Work out the finished part from the listing and answer in its coordinate system (mm). Face numbers are marked on the shaded views. A direction names the side the tool comes from. Round coordinates to 2 decimals unless told otherwise and drop trailing zeros. Write each loop counter-clockwise with the first axis right and the second up, starting at its lowest first coordinate (ties: lowest second). Pieces come first, ordered by that corner, then holes. Notation, with made-up numbers: (13.5, -18.5) - (24.5, -18.5) arc R23 cw to (24.5, 12.5) - close; hole circle Ø3 at (53, -20.5). An arc over 180 degrees is marked (long way). Answer as a JSON object with one key per item and string values.
```python
from build123d import *

# Parameters (mm, degrees)
F1_DEPTH = 254
F2_R     = 12.7
F4_D     = 12.7


with BuildPart() as f1:
    # F0 (on Front) → F1 (new body)
    with BuildSketch(Plane.XZ):
        Polygon((43.994091, 25.4), (0, 0), (381, 0), (1422.70971, 1041.70971), (1409.274401, 1067.10971), (367.564691, 25.4), align=None)
    extrude(amount=F1_DEPTH)

    # F2
    f2_edges = [f1.edges().sort_by_distance(p)[0] for p in [
        (367.564691, -127, 25.4),
    ]]
    fillet(f2_edges, radius=F2_R)

    # F4 (through all)
    with Locations(Plane(origin=(190.5, 0, -190.5), x_dir=(0, 1, 0), z_dir=(0.707107, 0, -0.707107))):
        with Locations((-203.2, 1412.407684), (-203.2, 1666.407684), (-50.8, 1666.407684), (-50.8, 1412.407684)):
            Hole(F4_D / 2)


solid = f1.part
```
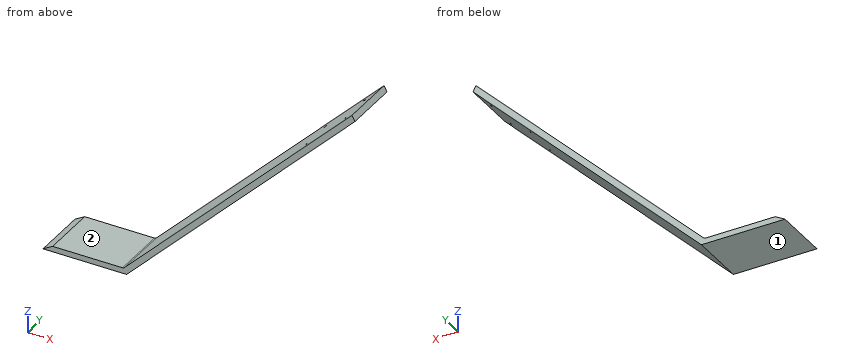
Item 1: A cutting plane is placed at A-A (y = -164). Write down the section's boundary in (x, z).
Results found:
{"outline": "(0, 0) - (381, 0) - (1422.71, 1041.71) - (1409.27, 1067.11) - (371.28, 29.12) arc R12.7 cw to (362.3, 25.4) - (43.99, 25.4) - close"}
Item 2: Each of these flat-tipped pins is pushed along its axis until it touches: P1, Ø4, axis at x = 823, y = -33, coming from the +Z side; P2, Ø8, axis at x = 843, y = -44, coming from the +Z side; P3, Ø5, axis at y = -153.5, z = 329.5, coming from the +X side. Where does it stop, or does it pass through?
Results found:
{"P1": "z = 482.84", "P2": "z = 504.84", "P3": "x = 713"}
Item 3: For the marked faces 1 and 2, determine the directions among +Z, -Z, +X, -X, +Y, -Y from which every point of the face is accessible in a straight line to the end or side of a thin tool.
Results found:
{"face 1": "-Z, +X, -X, +Y, -Y", "face 2": "+Z, -X, +Y, -Y"}
Item 4: A cutting plane is placed at C-C (z = 948.5). Write down the section's boundary in (x, y), and give its area (3 significant figures).
Results found:
{"outline": "(1290.66, -254) - (1329.5, -254) - (1329.5, 0) - (1290.66, 0) - close", "area": "9,860 mm²"}
Item 5: A cutting plane is placed at B-B (x = 325). Write down the section's boundary in (y, z).
Results found:
{"outline": "(-254, 0) - (0, 0) - (0, 25.4) - (-254, 25.4) - close"}
Item 6: Consider line 1 along Z through (x, y) = (209, -141); line 2 along Z through (x, y) = (364, -222); line 3 along X through (y, z) = (-116, 325). Determine where each line is inside the solid, lowest interval first.
Results found:
{"line 1": "0 to 25.4", "line 2": "0 to 25.51", "line 3": "667.16 to 706"}
